from build123d import *

# Parameters (mm, degrees)
SKETCH1_R           = 29
SKETCH1_R_2         = 25
SKETCH1_R_3         = 5
SKETCH1_R_4         = 3.5
BOSS_EXTRUDE3_DEPTH = 3.2


with BuildPart() as part:
    # Sketch1 → Boss-Extrude3 (new body)
    # profile 1 of 4: a face of its own
    with BuildSketch(Plane.XY):
        Circle(SKETCH1_R)
        Circle(SKETCH1_R_2, mode=Mode.SUBTRACT)
    # profile 2 of 4: a face of its own
    with BuildSketch(Plane.XY):
        with BuildLine():
            Line((18.29985715, 17.032769249), (3.65997143, 3.40655385))
            ThreePointArc((3.65997143, 3.40655385), (4.652948374, 1.830320034), (5, 0))
            Line((5, 0), (25, 0))
            ThreePointArc((25, 0), (23.264741872, 9.151600168), (18.29985715, 17.032769249))
        make_face()
    # profile 3 of 4: a face of its own
    with BuildSketch(Plane.XY):
        with BuildLine():
            ThreePointArc((-3.65997143, -3.40655385), (-4.652948374, -1.830320034), (-5, 0))
            Line((-5, 0), (-25, 0))
            ThreePointArc((-25, 0), (-23.264741872, -9.151600168), (-18.29985715, -17.032769249))
            Line((-18.29985715, -17.032769249), (-3.65997143, -3.40655385))
        make_face()
    # profile 4 of 4: a face of its own
    with BuildSketch(Plane.XY):
        Circle(SKETCH1_R_3)
        Circle(SKETCH1_R_4, mode=Mode.SUBTRACT)
    extrude(amount=BOSS_EXTRUDE3_DEPTH)

    # Sketch6 → Cut-Revolve4 (revolve, cut)
    with BuildSketch(Plane(origin=(0, 0, 0), x_dir=(0, 0, -1), z_dir=(1, 0, 0)), mode=Mode.PRIVATE) as cut_revolve4_sk:
        with BuildLine():
            Line((0, 29), (-3.2, 29))
            ThreePointArc((-3.2, 29), (-1.6, 27.4), (0, 29))
        make_face()
    revolve(cut_revolve4_sk.sketch.rotate(Axis((0, 0, 3.2), (0, 0, -1)), 90), axis=Axis((0, 0, 3.2), (0, 0, -1)), mode=Mode.SUBTRACT)


solid = part.part
Geometry check sheet. Reference: the model listing, model coordinates, mm. A direction names the side the tool comes from. Round coordinates to 2 decimals unless told otherwise and drop trailing zeros. Write each loop counter-clockwise with the first axis right and the second up, starting at its lowest first coordinate (ties: lowest second). Pieces come first, ordered by that corner, then holes. Notation, with made-up numbers: (14, -22) -> (68, -22) arc R20 cw to (68, 9) -> close; hole circle Ø1 at (12.25, -20). An arc over 180 degrees is marked (long way). One line per item, written item: value. Start each with the question number.
(1) Draft check along X on faces 1 (the flat face through (6, 0.4, 3.2)), 2 (the cylindrical face through (-1.752, 4.683, 1.578)). Enter one of: +X half, -X half, draft (parallel to the pull), parting line (faces both ways), or undercut.
(2) Go/stop test with flat-tipped pins: pin 1 Ø1.5 at (x, y) = (-10, 2.5) entering from +Z; pin 2 Ø1 at (x, z) = (-6.5, 1.5) entering from -Y; pin 3 Ø1.6 at (x, z) = (-17, 2) entering from +Y; pin 4 Ø1.5 at (x, z) = (-4, 2) entering from +Y. Record where each tip stops, or that it passes through.
(3) Cross-section at A-A, the plane x = 0. Record the cut outline in (y, z).
(4) Cross-section at C-C, the plane x = 9. Give the number of separate pieces and of enclosed holes in the cut face, and give its area (3 significant figures).
(5) Scan lines: line 1 (Y direction, x = 0, z = 1.45); line 2 (Y direction, x = 13, z = 2.6); line 3 (Y direction, x = 0, z = 1.15). Record each from-to range of solid material in increasing order. Write a range as [from, to].
(6) Access from +Z, -Z, +X, -X, +Y, -Y to the whole of each face (thin tool, end or side, straight path). Record for faces 3 (the cylindrical face through (8.8, -23.4, 1.6)), 4 (the flat face through (6, 0.4, 0)).
(7) Cross-section at B-B, the plane z = 1. Record the cut outline in (x, y).
Answer:
1. face 1: draft
1. face 2: undercut
2. pin 1: through
2. pin 2: y = -26.77
2. pin 3: y = 22.34
2. pin 4: y = 27.61
3. outline: (-29, 0) -> (-25, 0) -> (-25, 3.2) -> (-29, 3.2) arc R1.6 cw to start; (-5, 0) -> (-3.5, 0) -> (-3.5, 3.2) -> (-5, 3.2) -> close; (3.5, 0) -> (5, 0) -> (5, 3.2) -> (3.5, 3.2) -> close; (25, 0) -> (29, 0) arc R1.6 cw to (29, 3.2) -> (25, 3.2) -> close
4. separate pieces: 3
4. enclosed holes: 0
4. area: 45.5 mm²
5. line 1: [-27.41, -25], [-5, -3.5], [3.5, 5], [25, 27.41]
5. line 2: [-24.52, -21.35], [0, 12.1], [21.35, 24.52]
5. line 3: [-27.46, -25], [-5, -3.5], [3.5, 5], [25, 27.46]
6. face 3: +Z, -Z
6. face 4: -Z, +X, -X, +Y, -Y
7. outline: circle Ø55.03 at (0, 0); hole (-25, 0) -> (-5, 0) arc R5 cw to (3.66, 3.41) -> (18.3, 17.03) arc R25 ccw to start; hole (-18.3, -17.03) arc R25 ccw to (25, 0) -> (5, 0) arc R5 cw to (-3.66, -3.41) -> close; hole circle Ø7 at (0, 0)
